The listing builds one solid part. Answer for the finished solid, in the listing's coordinates (mm). A direction names the side the tool comes from. Give positions to 0.01 mm unless a question says otherwise; leave off trailing zeros. Write each loop counter-clockwise with the first axis right and the second up, starting at its lowest first coordinate (ties: lowest second). Pieces come first, ordered by that corner, then holes.
```python
from build123d import *

# Parameters (mm, degrees)
SKETCH2_W           = 101.6
SKETCH2_H           = 88.9
BOSS_EXTRUDE1_DEPTH = 3.175
SKETCH3_W           = 3.175
SKETCH3_H           = 88.9
BOSS_EXTRUDE2_DEPTH = 88.9
SKETCH5_R           = 1.524
SKETCH5_W           = 60.96
SKETCH5_H           = 63.5
CUT_EXTRUDE2_DEPTH  = 145.139405178
FILLET1_R           = 2.54
FILLET2_R           = 6.604
FILLET3_R           = 3.175
FILLET4_R           = 6.35
CUT_EXTRUDE3_DEPTH  = 143.132235964


with BuildPart() as part:
    # Sketch2 → Boss-Extrude1 (new body)
    with BuildSketch(Plane(origin=(0, 0, 0), x_dir=(1, 0, 0), z_dir=(0, 1, 0))):
        with Locations((50.8, 0)):
            Rectangle(SKETCH2_W, SKETCH2_H)
    extrude(amount=BOSS_EXTRUDE1_DEPTH)

    # Sketch3 → Boss-Extrude2 (add)
    with BuildSketch(Plane(origin=(0, 3.175, 0), x_dir=(1, 0, 0), z_dir=(0, 1, 0))):
        with Locations((100.0125, 0)):
            Rectangle(SKETCH3_W, SKETCH3_H)
    extrude(amount=BOSS_EXTRUDE2_DEPTH)

    # Sketch5 → Cut-Extrude2 (cut, through all)
    with BuildSketch(Plane(origin=(101.6, 0, 0), x_dir=(0, 0, -1), z_dir=(1, 0, 0))):
        with Locations((-37.973, 45.72)):
            Circle(SKETCH5_R)
        with Locations((37.973, 45.72)):
            Circle(SKETCH5_R)
        with Locations((0, 45.72)):
            Rectangle(SKETCH5_W, SKETCH5_H)
    extrude(amount=-CUT_EXTRUDE2_DEPTH, mode=Mode.SUBTRACT)

    # Fillet1
    fillet1_edges = [part.edges().sort_by_distance(p)[0] for p in [
        (100.0125, 13.97, 30.48),
        (100.0125, 77.47, 30.48),
        (100.0125, 77.47, -30.48),
        (100.0125, 13.97, -30.48),
    ]]
    fillet(fillet1_edges, radius=FILLET1_R)

    # Fillet2
    fillet2_edges = [part.edges().sort_by_distance(p)[0] for p in [
        (100.0125, 92.075, -44.45),
        (100.0125, 92.075, 44.45),
    ]]
    fillet(fillet2_edges, radius=FILLET2_R)

    # Fillet3
    fillet3_edges = [part.edges().sort_by_distance(p)[0] for p in [
        (98.425, 3.175, 0),
        (101.6, 0, 0),
    ]]
    fillet(fillet3_edges, radius=FILLET3_R)

    # Fillet4
    fillet4_edges = [part.edges().sort_by_distance(p)[0] for p in [
        (0, 1.5875, -44.45),
        (0, 1.5875, 44.45),
    ]]
    fillet(fillet4_edges, radius=FILLET4_R)

    # Sketch6 → Cut-Extrude3 (cut, through all)
    with BuildSketch(Plane(origin=(0, 3.175, 0), x_dir=(1, 0, 0), z_dir=(0, 1, 0))):
        with BuildLine():
            Line((17.795725812, 26.9875), (81.295725812, 26.9875))
            ThreePointArc((81.295725812, 26.9875), (82.883225812, 25.4), (81.295725812, 23.8125))
            Line((81.295725812, 23.8125), (17.795725812, 23.8125))
            ThreePointArc((17.795725812, 23.8125), (16.208225812, 25.4), (17.795725812, 26.9875))
        make_face()
        with BuildLine():
            Line((17.795725812, -26.9875), (81.295725812, -26.9875))
            ThreePointArc((81.295725812, -26.9875), (82.883225812, -25.4), (81.295725812, -23.8125))
            Line((81.295725812, -23.8125), (17.795725812, -23.8125))
            ThreePointArc((17.795725812, -23.8125), (16.208225812, -25.4), (17.795725812, -26.9875))
        make_face()
    extrude(amount=-CUT_EXTRUDE3_DEPTH, mode=Mode.SUBTRACT)


solid = part.part
```
Item 1: A cutting plane is placed at C-C, the plane y = 45.72. Give the vertices of the cut face in (x, z) (3 decimals), plus the area to 3 significant figures.
Conclusion:
outline: (98.425, -44.45) - (101.6, -44.45) - (101.6, -39.497) - (98.425, -39.497) - close; (98.425, -36.449) - (101.6, -36.449) - (101.6, -30.48) - (98.425, -30.48) - close; (98.425, 30.48) - (101.6, 30.48) - (101.6, 36.449) - (98.425, 36.449) - close; (98.425, 39.497) - (101.6, 39.497) - (101.6, 44.45) - (98.425, 44.45) - close
area: 69.4 mm2
Item 2: Consider probe 1 along Z at (x, y) = (100, 45); probe 2 along X at (y, z) = (10.5, -5) (3 decimals); probe 3 along Y at (x, z) = (70.5, 17.5) (3 decimals). Determine where each line is inside the solid, lowest interval first.
Conclusion:
probe 1: z = -44.45 to -39.32, -36.63 to -30.48, 30.48 to 36.63, 39.32 to 44.45
probe 2: x = 98.425 to 101.6
probe 3: y = 0 to 3.175
Item 3: A cutting plane is placed at D-D, the plane z = 9. Give the vertices of the cut face in (x, y) (3 decimals).
Conclusion:
outline: (0, 0) - (98.425, 0) arc R3.175 ccw to (101.6, 3.175) - (101.6, 13.97) - (98.425, 13.97) - (98.425, 6.35) arc R3.175 cw to (95.25, 3.175) - (0, 3.175) - close; (98.425, 77.47) - (101.6, 77.47) - (101.6, 92.075) - (98.425, 92.075) - close
Item 4: A cutting plane is placed at A-A, the plane x = 37. Count the separate pieces of the cut face and the enclosed holes in it, plus the area to 3 significant figures.
Conclusion:
separate pieces: 3
enclosed holes: 0
area: 262 mm2
Item 5: Each of these flat-tipped pins is pushed along its axis until it touches: P1, Ø2.5, axis at x = 100.5, z = -7.5, coming from the -Y side; P2, Ø4, axis at x = 43, z = 9, coming from the +Y side (3 decimals); P3, Ø3.5, axis at y = 45.72, z = 37.973, coming from the -X side (3 decimals); P4, Ø10, axis at x = 70.5, z = -5.5, coming from the -Y side. Where does it stop, or does it pass through?
Conclusion:
P1: stops at y = 0.11
P2: stops at y = 3.175
P3: stops at x = 98.425
P4: stops at y = 0
Item 6: Determine the mould class of faces 6 (the face through (99.99, 76.746, -29.716)), 7 (the face through (97.52, 4.13, -0.62)), 8 (the face through (100.035, 90.192, -42.464)) for opening direction Z: pulls with the +Z half, pulls with the -Z half, needs draft (parallel to the pull), parting line crosses it, or undercut.
Conclusion:
face 6: undercut
face 7: needs draft
face 8: pulls with the -Z half
Item 7: A cutting plane is placed at B-B, the plane z = 25.4. Give the vertices of the cut face in (x, y) (3 decimals), plus the area to 3 significant figures.
Conclusion:
outline: (0, 0) - (16.208, 0) - (16.208, 3.175) - (0, 3.175) - close; (82.883, 0) - (98.425, 0) arc R3.175 ccw to (101.6, 3.175) - (101.6, 13.97) - (98.425, 13.97) - (98.425, 6.35) arc R3.175 cw to (95.25, 3.175) - (82.883, 3.175) - close; (98.425, 77.47) - (101.6, 77.47) - (101.6, 92.075) - (98.425, 92.075) - close
area: 192 mm2
Item 8: Which of the six approach directions +Z, -Z, +X, -X, +Y, -Y give full straight-line access (tool end or side, diameter ignored) to faces 1 (the face through (16.21, 1.61, 25.37)), 2 (the face through (100.035, 90.089, 42.567)), 3 (the face through (100, 45, -30.48)), 4 (the face through (47, 3.175, -1)), 5 (the face through (1.91, 1.61, 42.64))?
Conclusion:
face 1: +Y, -Y
face 2: +Z, +X, -X, +Y
face 3: +X, -X
face 4: +Z, -Z, -X, +Y
face 5: +Z, -X, +Y, -Y
